Here's the drawing with two shaded views (mm, measured from the low corner). I have some questions. A direction names the side the tool comes from. Give positions to 0.01 mm unless a question says otherwise; leave off trailing zeros. Loops run counter-clockwise (first coordinate to the right, second up) from the corner with the lowest first, then second, coordinate; pieces in that order, holes last. Notation, with made-up numbers: (89.25, 67) -> (96.25, 67) arc R21 ccw to (96.25, 75) -> close; hole circle Ø7 at (-20, 70). An arc over 180 degrees is marked (long way). Answer in a Markdown table with one row per item. Add a question column.
Item 1: If we section it at B-B (z = 5.75): Write out the boundary of the cut face in (x, y), then the cut area to 3 significant figures.
Item 2: If we section it at D-D (y = 22.86): Write out the boundary of the cut face in (x, z), then the cut area to 3 significant figures.
Item 3: For P1, Ø2.5, axis at x = 56.5, z = 2.5, coming from the +Y side; P2, Ø2.5, axis at x = 37, z = 14, coming from the -Y side; P3, Ø3.5, axis at x = 21.336, y = 22.86, coming from the -Z side, each with a flat end and sliding along its axis, tell me the tip position at first contact or that it passes through.
Item 4: If I drill on line 1 (X direction, y = 3.25, z = 11.5); line 2 (Y direction, x = 38, z = 11.5); line 3 (Z direction, x = 61, y = 10), over which ranges is the centre line in solid material (lowest first)?
Item 5: We'd pull the mould along X, two halves only. Please class the marked faces 4, 5 and 6: released by +X, released by -X, zero draft, split by the parting line, or undercut.
Item 6: If we section it at C-C (x = 5.08): Write out the boundary of the cut face in (y, z), then the cut area to 3 significant figures.
Item 7: If we section it at A-A (y = 2.75): Write out the boundary of the cut face in (x, z).
Item 8: Which directions (+Z, -Z, +X, -X, +Y, -Y) give clear straight access to the entire face, cutting with the end or side of a thin tool? Please do the marked faces 1, 2 and 3.
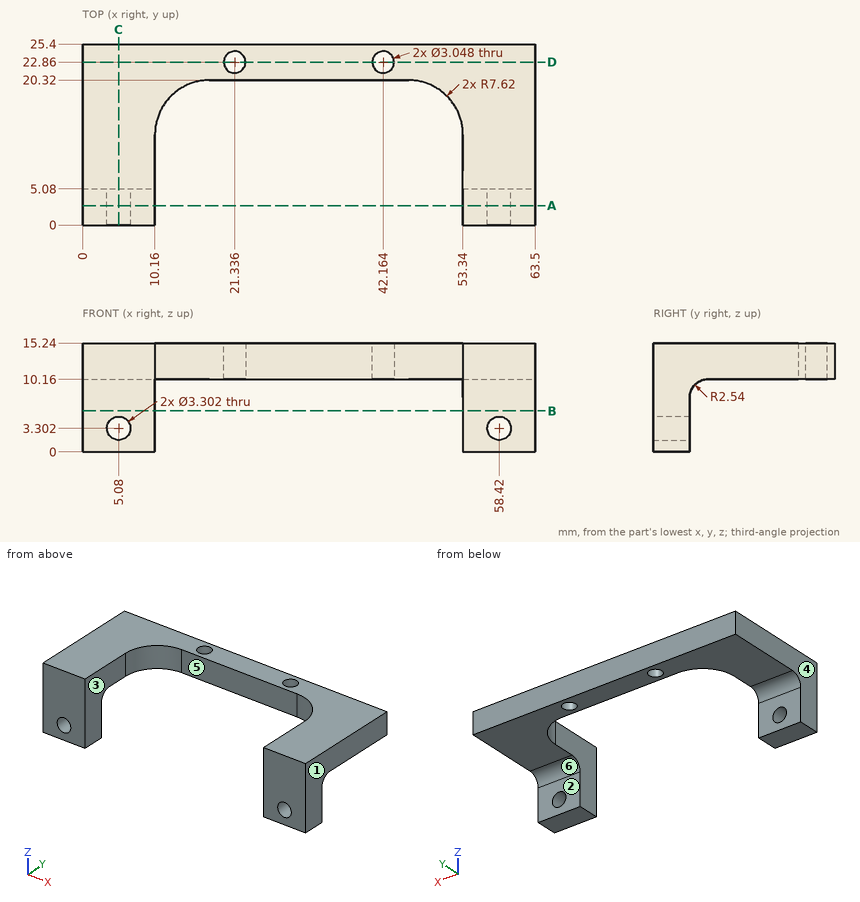
Recorded:
| question | item | result |
|---|---|---|
| 1 | outline | (0, 0) -> (10.16, 0) -> (10.16, 5.08) -> (0, 5.08) -> close; (53.34, 0) -> (63.5, 0) -> (63.5, 5.08) -> (53.34, 5.08) -> close |
| 1 | area | 103 mm^2 |
| 2 | outline | (0, 10.16) -> (19.81, 10.16) -> (19.81, 15.24) -> (0, 15.24) -> close; (22.86, 10.16) -> (40.64, 10.16) -> (40.64, 15.24) -> (22.86, 15.24) -> close; (43.69, 10.16) -> (63.5, 10.16) -> (63.5, 15.24) -> (43.69, 15.24) -> close |
| 2 | area | 292 mm^2 |
| 3 | P1 | stops at y = 5.08 |
| 3 | P2 | stops at y = 20.32 |
| 3 | P3 | stops at z = 10.16 |
| 4 | line 1 | x = 0 to 10.16, 53.34 to 63.5 |
| 4 | line 2 | y = 20.32 to 25.4 |
| 4 | line 3 | z = 10.16 to 15.24 |
| 5 | face 4 | released by -X |
| 5 | face 5 | undercut |
| 5 | face 6 | zero draft |
| 6 | outline | (0, 0) -> (5.08, 0) -> (5.08, 1.65) -> (0, 1.65) -> close; (0, 4.95) -> (5.08, 4.95) -> (5.08, 7.62) arc R2.54 cw to (7.62, 10.16) -> (25.4, 10.16) -> (25.4, 15.24) -> (0, 15.24) -> close |
| 6 | area | 165 mm^2 |
| 7 | outline | (0, 0) -> (10.16, 0) -> (10.16, 15.24) -> (0, 15.24) -> close; (53.34, 0) -> (63.5, 0) -> (63.5, 15.24) -> (53.34, 15.24) -> close; hole circle Ø3.3 at (5.08, 3.3); hole circle Ø3.3 at (58.42, 3.3) |
| 8 | face 1 | +Z, -Z, +X, +Y, -Y |
| 8 | face 2 | -Z, +X, -X, +Y |
| 8 | face 3 | +Z, -Z, -Y |
